```python
from build123d import *

# Parameters (mm, degrees)
F1_DEPTH = 57.15
F0_W     = 57.912
F0_H     = 26.162
F2_DEPTH = 44.45
F3_SIZE2 = 3.175
F3_SIZE  = 0.8128
F4_R     = 1.5748


with BuildPart() as f1:
    # F0 (on Top) → F1 (new body)
    with BuildSketch(Plane.XY):
        with BuildLine():
            Line((29.4132, 17.526), (-29.4132, 17.526))
            ThreePointArc((-29.4132, 17.526), (-32.233000422, 16.358000422), (-33.401, 13.5382))
            Line((-33.401, 13.5382), (-33.401, -13.5382))
            ThreePointArc((-33.401, -13.5382), (-32.233000422, -16.358000422), (-29.4132, -17.526))
            Line((-29.4132, -17.526), (29.4132, -17.526))
            ThreePointArc((29.4132, -17.526), (32.233000422, -16.358000422), (33.401, -13.5382))
            Line((33.401, -13.5382), (33.401, 13.5382))
            ThreePointArc((33.401, 13.5382), (32.233000422, 16.358000422), (29.4132, 17.526))
        make_face()
        with BuildLine():
            Line((-29.4132, 14.351), (29.4132, 14.351))
            ThreePointArc((29.4132, 14.351), (29.9879363917, 14.1129363917), (30.226, 13.5382))
            Line((30.226, 13.5382), (30.226, -13.5382))
            ThreePointArc((30.226, -13.5382), (29.9879363917, -14.1129363917), (29.4132, -14.351))
            Line((29.4132, -14.351), (-29.4132, -14.351))
            ThreePointArc((-29.4132, -14.351), (-29.9879363917, -14.1129363917), (-30.226, -13.5382))
            Line((-30.226, -13.5382), (-30.226, 13.5382))
            ThreePointArc((-30.226, 13.5382), (-29.9879363917, 14.1129363917), (-29.4132, 14.351))
        make_face(mode=Mode.SUBTRACT)
    extrude(amount=F1_DEPTH)

    # F0 (on Top) → F2 (join)
    with BuildSketch(Plane.XY):
        with BuildLine():
            ThreePointArc((30.226, 13.5382), (29.9879363917, 14.1129363917), (29.4132, 14.351))
            Line((29.4132, 14.351), (-29.4132, 14.351))
            ThreePointArc((-29.4132, 14.351), (-29.9879363917, 14.1129363917), (-30.226, 13.5382))
            Line((-30.226, 13.5382), (-30.226, -13.5382))
            ThreePointArc((-30.226, -13.5382), (-29.9879363917, -14.1129363917), (-29.4132, -14.351))
            Line((-29.4132, -14.351), (29.4132, -14.351))
            ThreePointArc((29.4132, -14.351), (29.9879363917, -14.1129363917), (30.226, -13.5382))
            Line((30.226, -13.5382), (30.226, 13.5382))
        make_face()
        Rectangle(F0_W, F0_H, mode=Mode.SUBTRACT)
    extrude(amount=F2_DEPTH)

    # F3
    f3_edges = [f1.edges().sort_by_distance(p)[0] for p in [
        (0, 17.526, 57.15),
        (-32.233, 16.358, 57.15),
        (-33.401, 0, 57.15),
        (-32.233, -16.358, 57.15),
        (0, -17.526, 57.15),
        (32.233, -16.358, 57.15),
        (33.401, 0, 57.15),
        (32.233, 16.358, 57.15),
        (0, 14.351, 57.15),
        (29.987936, 14.112936, 57.15),
        (30.226, 0, 57.15),
        (29.987936, -14.112936, 57.15),
        (0, -14.351, 57.15),
        (-29.987936, -14.112936, 57.15),
        (-30.226, 0, 57.15),
        (-29.987936, 14.112936, 57.15),
    ]]
    f3_side = f1.faces().sort_by_distance((0, 16.771603, 57.15))[0]
    chamfer(f3_edges, length=F3_SIZE, length2=F3_SIZE2, reference=f3_side)

    # F4
    f4_edges = [f1.edges().sort_by_distance(p)[0] for p in [
        (0, 17.526, 0),
        (-32.233, 16.358, 0),
        (-33.401, 0, 0),
        (-32.233, -16.358, 0),
        (0, -17.526, 0),
        (32.233, -16.358, 0),
        (33.401, 0, 0),
        (32.233, 16.358, 0),
        (0, -13.081, 0),
        (-28.956, 0, 0),
        (0, 13.081, 0),
        (28.956, 0, 0),
    ]]
    fillet(f4_edges, radius=F4_R)


solid = f1.part
```
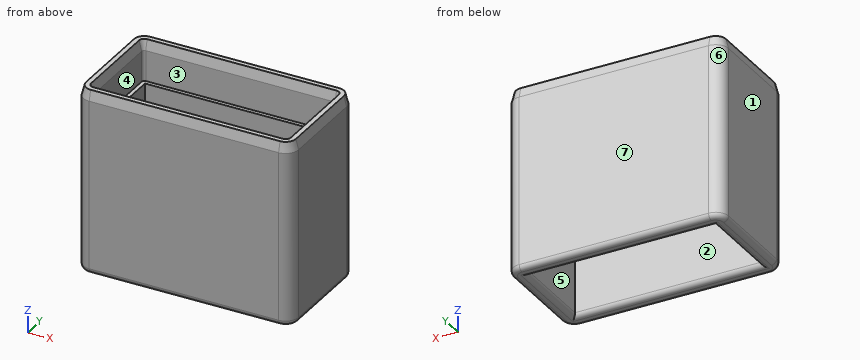
The model under review builds one solid part; all positions refer to its coordinate system, in mm. Face numbers are marked on the shaded views. A direction names the side the tool comes from. Round coordinates to 2 decimals unless told otherwise and drop trailing zeros. Loops run counter-clockwise (first coordinate to the right, second up) from the corner with the lowest first, then second, coordinate; pieces in that order, holes last. Notation, with made-up numbers: (-17.5, -22) -> (-12.5, -22) arc R31 cw to (-12.5, 17) -> close; hole circle Ø10 at (89, 57). An arc over 180 degrees is marked (long way). Answer as a JSON object with one key per item and string values. Group by question number.
1) We need section A-A on y = -6.5. Write out the cut boundary in (x, z) (3 decimals).
2) For pin 1 Ø12 at (x, y) = (9, 5) entering from -Z, flat-tipped, find the tip position at first contact; note if it passes through.
3) Mouldability with a two-part tool opening along X and no side actions: class the marked faces 4, 5, 6 and 7 as released by +X, released by -X, zero draft, split by the parting line, or undercut.
4) We need section C-C on x = -21.5. Write out the cut boundary in (y, z) (3 decimals).
5) We need section D-D on z = 46. Write out the cut boundary in (x, y).
6) For line 1 (X direction, y = 1, z = 16.5); line 2 (Y direction, x = -15, z = 42); line 3 (Y direction, x = 28, z = 47.5), list the stretches that pass through material, from the lowest coordinate up. Write a range as [from, to].
7) We need section B-B on z = 5. Write out the cut boundary in (x, y).
8) For the marked faces 1, 2 and 3, list the 3-axis set-ups (+Z, -Z, +X, -X, +Y, -Y) from which the entire face can be reached by the end or side of a thin tool; tool diameter is ignored.
Result set:
{
 "1": {"outline": "(-33.401, 1.575) arc R1.575 ccw to (-31.826, 0) -> (-30.531, 0) arc R1.575 ccw to (-28.956, 1.575) -> (-28.956, 44.45) -> (-30.226, 44.45) -> (-30.226, 53.975) -> (-31.039, 57.15) -> (-32.588, 57.15) -> (-33.401, 53.975) -> close; (28.956, 1.575) arc R1.575 ccw to (30.531, 0) -> (31.826, 0) arc R1.575 ccw to (33.401, 1.575) -> (33.401, 53.975) -> (32.588, 57.15) -> (31.039, 57.15) -> (30.226, 53.975) -> (30.226, 44.45) -> (28.956, 44.45) -> close"},
 "2": {"pin 1": "through"},
 "3": {"face 4": "undercut", "face 5": "undercut", "face 6": "released by -X", "face 7": "zero draft"},
 "4": {"outline": "(-17.526, 1.575) arc R1.575 ccw to (-15.951, 0) -> (-14.656, 0) arc R1.575 ccw to (-13.081, 1.575) -> (-13.081, 44.45) -> (-14.351, 44.45) -> (-14.351, 53.975) -> (-15.164, 57.15) -> (-16.713, 57.15) -> (-17.526, 53.975) -> close; (13.081, 1.575) arc R1.575 ccw to (14.656, 0) -> (15.951, 0) arc R1.575 ccw to (17.526, 1.575) -> (17.526, 53.975) -> (16.713, 57.15) -> (15.164, 57.15) -> (14.351, 53.975) -> (14.351, 44.45) -> (13.081, 44.45) -> close"},
 "5": {"outline": "(-33.4, -13.54) arc R3.99 ccw to (-29.41, -17.53) -> (29.41, -17.53) arc R3.99 ccw to (33.4, -13.54) -> (33.4, 13.54) arc R3.99 ccw to (29.41, 17.53) -> (-29.41, 17.53) arc R3.99 ccw to (-33.4, 13.54) -> close; hole (-30.23, -13.54) arc R0.81 ccw to (-29.41, -14.35) -> (29.41, -14.35) arc R0.81 ccw to (30.23, -13.54) -> (30.23, 13.54) arc R0.81 ccw to (29.41, 14.35) -> (-29.41, 14.35) arc R0.81 ccw to (-30.23, 13.54) -> close"},
 "6": {"line 1": "[-33.4, -28.96], [28.96, 33.4]", "line 2": "[-17.53, -13.08], [13.08, 17.53]", "line 3": "[-17.53, -14.35], [14.35, 17.53]"},
 "7": {"outline": "(-33.4, -13.54) arc R3.99 ccw to (-29.41, -17.53) -> (29.41, -17.53) arc R3.99 ccw to (33.4, -13.54) -> (33.4, 13.54) arc R3.99 ccw to (29.41, 17.53) -> (-29.41, 17.53) arc R3.99 ccw to (-33.4, 13.54) -> close; hole (-28.96, -13.08) -> (28.96, -13.08) -> (28.96, 13.08) -> (-28.96, 13.08) -> close"},
 "8": {"face 1": "+Z, -Z, -X, +Y, -Y", "face 2": "+Z, -Z", "face 3": "+Z"}
}
